Part model, mm, in its own coordinate system. A direction names the side the tool comes from. Give positions to 0.01 mm unless a question says otherwise; leave off trailing zeros. Write each loop counter-clockwise with the first axis right and the second up, starting at its lowest first coordinate (ties: lowest second). Pieces come first, ordered by that corner, then holes. Notation, with made-up numbers: M -25.75,36.5 L -7.75,36.5 A14 cw -7.75,56.5 Z; hole C 35.25,-22 d7. An arc over 180 degrees is marked long. Answer as CSV lines item,"result". Start each with the question number.
Item 1: Wall check: L1, parallel to Y at x = 57.5, z = 2.25; L2, parallel to Z at x = 11, y = -33; L3, parallel to Y at x = 33.5, z = 15. Give the ranges that are in metal, low to high. Write a range as from..to.
Item 2: Band-saw the part on B-B, the plane z = 12. List the corners of the cut face in (x, y), then the cut area to 4 significant figures.
Item 3: Band-saw the part on A-A, the plane x = 52.5. List the corners of the cut face in (y, z), then the cut area to 3 significant figures.
Item 4: Band-saw the part on C-C, the plane x = 21.5. List the corners of the cut face in (y, z).
Item 5: Two-plate mould, pull along Y, no slides. Class faces 4 (the flat face through (32, 19.44, 15)), 5 (the cylindrical face through (61.825, 15.921, 14.232)), 6 (the flat face through (63, -35, 2)): +Y half, -Y half, draft (parallel to the pull), parting line (faces both ways), or undercut.
Item 6: Band-saw the part on D-D, the plane y = -17. List the corners of the cut face in (x, z), then the cut area to 4 significant figures.
Item 7: 3-axis set-ups, long thin cutter, end or side, ignore diameter. For faces 1 (the flat face through (2, 17, 13)), 2 (the flat face through (8, -35, 6)), 3 (the flat face through (4.75, -35, 1)): which of +Z, -Z, +X, -X, +Y, -Y reach the whole face in a straight line?
Item 8: Pin check, flat tips, straight feed: pin 1 (4 mm diameter, centred on x = 64, y = 17.5, fed in from -Z); pin 2 (0.8 mm diameter, centred on y = 17, z = 13.5, fed in from +X); pin 3 (1.5 mm diameter, centred on x = 39, z = 4.5, fed in from +Y). Stop position of each tip, or through.
from build123d import *

# Parameters (mm, degrees)
F1_DEPTH = 65.5
F2_R     = 5
F4_DEPTH = 1
F6_D     = 1.5
F6_DEPTH = 5
F7_W     = 15
F7_H     = 7
F7_W_2   = 8
F7_H_2   = 4
F8_DEPTH = 5
F7_W_3   = 4.75
F7_H_3   = 2
F9_DEPTH = 5


with BuildPart() as f1:
    # F0 (on Right) → F1 (new body)
    with BuildSketch(Plane.YZ):
        with BuildLine():
            Line((-36.059797, 0), (-34.559797, 0))
            Line((-34.559797, 0), (-34.559797, 14))
            Line((-34.559797, 14), (19.440203, 14))
            Line((19.440203, 14), (19.440203, 15.5))
            Line((19.440203, 15.5), (-34.059797, 15.5))
            ThreePointArc((-34.059797, 15.5), (-35.47401, 14.914214), (-36.059797, 13.5))
            Line((-36.059797, 13.5), (-36.059797, 0))
        make_face()
    extrude(amount=F1_DEPTH)

    # F2
    f2_edges = [f1.edges().sort_by_distance(p)[0] for p in [
        (65.5, 19.440203, 14.75),
        (0, 19.440203, 14.75),
    ]]
    fillet(f2_edges, radius=F2_R)

    # F3 (on face) → F4 (join)
    with BuildSketch(Plane(origin=(0, 0, 14), x_dir=(1, 0, 0), z_dir=(0, 0, -1))):
        with BuildLine():
            ThreePointArc((0, -14.440203), (1.464466, -17.975737), (5, -19.440203))
            Line((5, -19.440203), (5, -14.440203))
            Line((5, -14.440203), (0, -14.440203))
        make_face()
        with BuildLine():
            ThreePointArc((60.5, -19.440203), (64.035534, -17.975737), (65.5, -14.440203))
            Line((65.5, -14.440203), (60.5, -14.440203))
            Line((60.5, -14.440203), (60.5, -19.440203))
        make_face()
    extrude(amount=F4_DEPTH)

    # F6
    with Locations(Plane.XY.offset(15.5)):
        with Locations((2.982233, 16.20797), (62.517767, 16.20797)):
            Hole(F6_D / 2, depth=F6_DEPTH)

    # F7 (on face) → F8 (cut)
    with BuildSketch(Plane.XZ.offset(36.059797)):
        with Locations((54, 9.5)):
            Rectangle(F7_W, F7_H)
        with Locations((12, 6.5)):
            Rectangle(F7_W_2, F7_H_2)
    extrude(amount=-F8_DEPTH, mode=Mode.SUBTRACT)

    # F7 (on face) → F9 (cut)
    with BuildSketch(Plane.XZ.offset(36.059797)):
        with Locations((2.375, 1)):
            Rectangle(F7_W_3, F7_H_3)
        with Locations((63.125, 1)):
            Rectangle(F7_W_3, F7_H_3)
    extrude(amount=-F9_DEPTH, mode=Mode.SUBTRACT)


solid = f1.part
Output:
1,L1,"-36.06..-34.56"
1,L2,"14..15.5"
1,L3,"-35.38..19.44"
2,outline,"M 0,-36.06 L 46.5,-36.06 L 46.5,-34.56 L 0,-34.56 Z; M 61.5,-36.06 L 65.5,-36.06 L 65.5,-34.56 L 61.5,-34.56 Z"
2,area,"75.75 mm²"
3,outline,"M -36.06,0 L -34.56,0 L -34.56,6 L -36.06,6 Z; M -36.06,13 L -34.56,13 L -34.56,14 L 19.44,14 L 19.44,15.5 L -34.06,15.5 A2 ccw -36.06,13.5 Z"
3,area,"92.9 mm²"
4,outline,"M -36.06,0 L -34.56,0 L -34.56,14 L 19.44,14 L 19.44,15.5 L -34.06,15.5 A2 ccw -36.06,13.5 Z"
5,face 4,"+Y half"
5,face 5,"undercut"
5,face 6,"draft"
6,outline,"M 0,14 L 65.5,14 L 65.5,15.5 L 0,15.5 Z"
6,area,"98.25 mm²"
7,face 1,"-Z, +X, -X, +Y"
7,face 2,"+Y, -Y"
7,face 3,"-Z, -X, +Y, -Y"
8,pin 1,"z = 13"
8,pin 2,"x = 65.01"
8,pin 3,"y = -34.56"
